```python
from build123d import *

# Parameters (mm, degrees)
F1_W      = 59.69
F1_H      = 28.575
F1_R      = 1.5748
F1_R_2    = 0.79375
F2_DEPTH  = 2.54
F3_W      = 5.600192
F3_H      = 7.500214
F4_DEPTH  = 2.54
F5_W      = 16.800018
F5_H      = 3.139999
F6_DEPTH  = 2.921
F7_W      = 4.826
F7_H      = 2.4892
F7_W_2    = 4.2418
F7_H_2    = 3.2512
F8_DEPTH  = 2.286
F9_R      = 0.4445
F10_DEPTH = 6.096


with BuildPart() as f2:
    # F1 (on Top) → F2 (new body)
    with BuildSketch(Plane.XY):
        with Locations((-0.701548, 0)):
            Rectangle(F1_W, F1_H)
        with Locations((-27.371548, -11.2395)):
            Circle(F1_R, mode=Mode.SUBTRACT)
        with Locations((9.331452, -9.4615)):
            Circle(F1_R_2, mode=Mode.SUBTRACT)
        with Locations((14.538452, -11.2395)):
            Circle(F1_R, mode=Mode.SUBTRACT)
        with Locations((-27.371548, 11.1125)):
            Circle(F1_R, mode=Mode.SUBTRACT)
        with Locations((-19.370548, 11.1125)):
            Circle(F1_R_2, mode=Mode.SUBTRACT)
        with Locations((14.538452, 11.1125)):
            Circle(F1_R, mode=Mode.SUBTRACT)
    extrude(amount=F2_DEPTH)

    # F3 (on face) → F4 (join)
    with BuildSketch(Plane.XY.offset(2.54)):
        with Locations((27.619452, 8.8265)):
            Rectangle(F3_W, F3_H)
        with Locations((27.746452, -3.6195)):
            Rectangle(F3_W, F3_H)
    extrude(amount=F4_DEPTH)

    # F5 (on face) → F6 (join)
    with BuildSketch(Plane.XY.offset(2.54)):
        with Locations((-1.058545, -8.963304)):
            Rectangle(F5_W, F5_H)
    extrude(amount=F6_DEPTH)

    # F7 (on face) → F8 (join)
    with BuildSketch(Plane.XY.offset(2.54)):
        with Locations((26.349452, -11.4935)):
            Rectangle(F7_W, F7_H)
        with Locations((-27.244548, 6.2865)):
            Rectangle(F7_W, F7_H)
        with Locations((-27.117548, 2.4765)):
            Rectangle(F7_W, F7_H)
        with Locations((-27.117548, -5.9055)):
            Rectangle(F7_W_2, F7_H_2)
    extrude(amount=F8_DEPTH)

    # F9 (on face) → F10 (join)
    with BuildSketch(Plane.XY.offset(4.826)):
        with Locations((-28.514548, 6.2865)):
            Circle(F9_R)
        with Locations((-25.974548, 6.2865)):
            Circle(F9_R)
        with Locations((-28.387548, 2.4765)):
            Circle(F9_R)
        with Locations((-25.974548, 2.4765)):
            Circle(F9_R)
        with Locations((27.619452, -11.4935)):
            Circle(F9_R)
        with Locations((25.079452, -11.4935)):
            Circle(F9_R)
    extrude(amount=F10_DEPTH)


solid = f2.part
```
Verification items for the finished model (mm, model axes). A direction names the side the tool comes from. Coordinates: 2 decimals unless noted, no trailing zeros. Loops run counter-clockwise (first coordinate to the right, second up) from the corner with the lowest first, then second, coordinate; pieces in that order, holes last. Notation, with made-up numbers: (22, 12) - (72, 12) arc R13 cw to (72, 20) - close; hole circle Ø9 at (-24.75, -30). An arc over 180 degrees is marked (long way). Put each result on its own line as item: value.
Item 1: Gauge pin test, flat ends, axial feed: pin 1 Ø0.8 at (y, z) = (7, 3.5) entering from +X; pin 2 Ø1.1 at (y, z) = (3, 3.5) entering from -X; pin 3 Ø1.8 at (x, z) = (-27, 4) entering from +Y; pin 4 Ø1 at (x, z) = (9, 5) entering from +Y. Record the tip position at first contact, or that the pin passes through.
Conclusion:
pin 1: stops at x = 30.42
pin 2: stops at x = -29.53
pin 3: stops at y = 7.53
pin 4: passes through
Item 2: Set-up check for faces 1 (the face through (-27, 6, 4.826)), 2 (the face through (-27, 5.042, 4)), 3 (the face through (30, 9, 2.54)), 4 (the face through (-27, -7.531, 4)): record each of +Z, -Z, +X, -X, +Y, -Y from which the full face is reachable in a straight line by a thin tool's end or side.
Conclusion:
face 1: +Z
face 2: +Z, +X, -X
face 3: -Z, +X, +Y, -Y
face 4: +Z, -X, -Y
Item 3: Draft check along X on faces 5 (the face through (15.27, 9.72, 1.25)), 6 (the face through (-30.547, 0, 1)), 7 (the face through (30.42, 9, 4)). Enter one of: pulls with the +X half, pulls with the -X half, needs draft (parallel to the pull), parting line crosses it, or undercut.
Conclusion:
face 5: undercut
face 6: pulls with the -X half
face 7: pulls with the +X half
Item 4: Section check D-D (z = 1). Enter the section's corners in (x, y), then the cut area to 3 significant figures.
Conclusion:
outline: (-30.55, -14.29) - (29.14, -14.29) - (29.14, 14.29) - (-30.55, 14.29) - close; hole circle Ø3.15 at (-27.37, -11.24); hole circle Ø3.15 at (-27.37, 11.11); hole circle Ø1.59 at (-19.37, 11.11); hole circle Ø1.59 at (9.33, -9.46); hole circle Ø3.15 at (14.54, -11.24); hole circle Ø3.15 at (14.54, 11.11)
area: 1,670 mm2
Item 5: Scan lines: line 1 along X through (y, z) = (10, 2.25); line 2 along Z through (x, y) = (10, 11); line 3 along Z through (x, y) = (-2, -8.5). Record each from-to range of solid material in increasing order.
Conclusion:
line 1: x = -30.55 to -28.49, -26.26 to 13.42, 15.65 to 29.14
line 2: z = 0 to 2.54
line 3: z = 0 to 5.46
Item 6: Section check C-C (x = -3). Enter the section's corners in (y, z), then the cut area to 3 significant figures.
Conclusion:
outline: (-14.29, 0) - (14.29, 0) - (14.29, 2.54) - (-7.39, 2.54) - (-7.39, 5.46) - (-10.53, 5.46) - (-10.53, 2.54) - (-14.29, 2.54) - close
area: 81.8 mm2
Item 7: Section check B-B (y = -3). Enter the section's corners in (x, z).
Conclusion:
outline: (-30.55, 0) - (29.14, 0) - (29.14, 2.54) - (30.55, 2.54) - (30.55, 5.08) - (24.95, 5.08) - (24.95, 2.54) - (-30.55, 2.54) - close
Item 8: Section check A-A (z = 3.5). Enter the section's corners in (x, y), then the cut area to 3 significant figures.
Conclusion:
outline: (-29.66, 5.04) - (-24.83, 5.04) - (-24.83, 7.53) - (-29.66, 7.53) - close; (-29.53, 1.23) - (-24.7, 1.23) - (-24.7, 3.72) - (-29.53, 3.72) - close; (-29.24, -7.53) - (-25, -7.53) - (-25, -4.28) - (-29.24, -4.28) - close; (-9.46, -10.53) - (7.34, -10.53) - (7.34, -7.39) - (-9.46, -7.39) - close; (23.94, -12.74) - (28.76, -12.74) - (28.76, -10.25) - (23.94, -10.25) - close; (24.82, 5.08) - (30.42, 5.08) - (30.42, 12.58) - (24.82, 12.58) - close; (24.95, -7.37) - (30.55, -7.37) - (30.55, 0.13) - (24.95, 0.13) - close
area: 187 mm2
